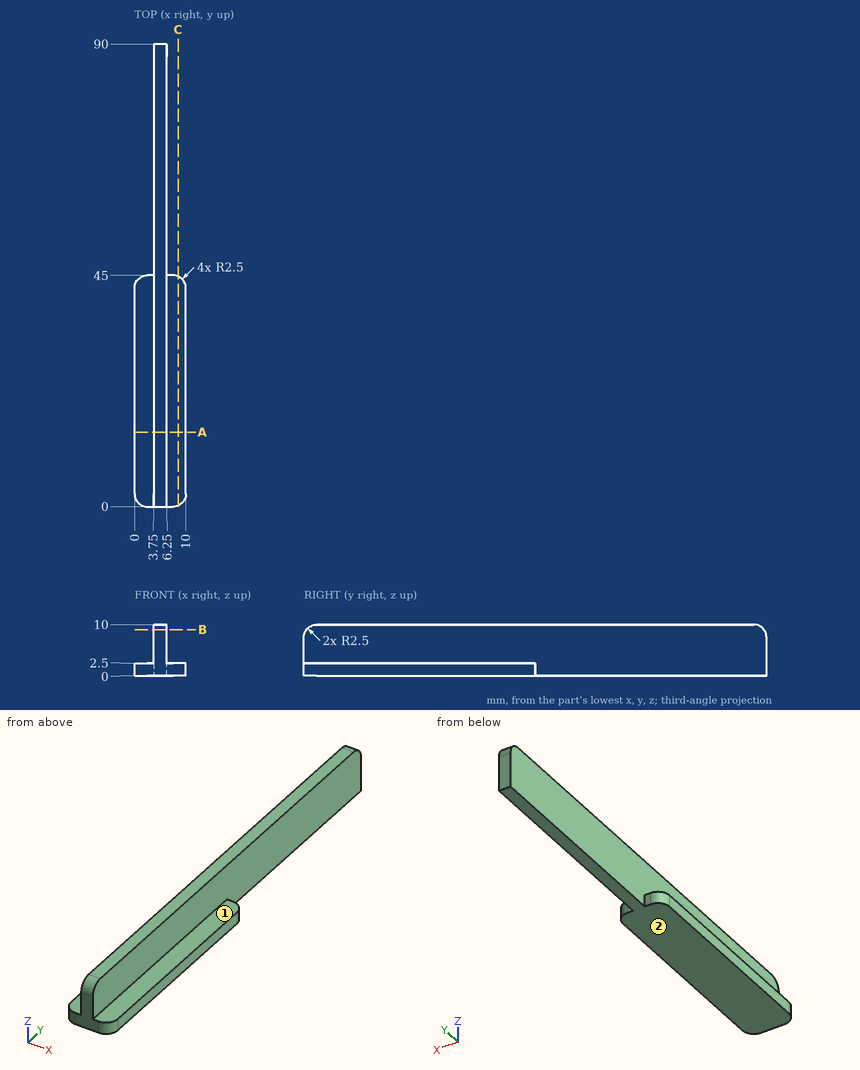
Geometry: see drawing. Coordinates: mm, zero at the bounding-box minimum. A direction names the side the tool comes from. Give positions to 0.01 mm unless a question says otherwise; leave off trailing zeros. Write each loop counter-clockwise with the first axis right and the second up, starting at its lowest first coordinate (ties: lowest second). Pieces come first, ordered by that corner, then holes. Notation, with made-up numbers: M -5.5,10 L 24.5,10 A26 cw 24.5,24 Z; hole C -8,55.25 d1. An arc over 180 degrees is marked long. Answer in a Markdown table with one row per item. Add a question column.
(1) Section B-B on z = 9. Return loops of the section in (x, y), and give its area (4 significant figures).
(2) Reachability of the marked faces 1 and 2 from +Z, -Z, +X, -X, +Y, -Y: full face, straight path, thin tool, end or side. Return the list, or none.
(3) Section C-C on x = 8.5. Return loops of the section in (y, z), and give its area (3 significant figures).
(4) First-contact query: pin 1 (1 mm diameter, centred on x = 3, z = 1, fed in from +Y); pin 2 (4 mm diameter, centred on x = 1.5, y = 12, fed in from +Z). Flat tips, straight axial feed; report the tip coordinate or a pass-through.
(5) Ray query, line 1 (X direction, y = 84, z = 2); line 2 (Y direction, x = 6, z = 8.5). Return the intervals inside material, ascending.
(6) Section A-A on y = 14.5. Return loops of the section in (x, z), and give its area (4 significant figures).
Result set:
| question | item | result |
|---|---|---|
| 1 | outline | M 3.75,0.5 L 6.25,0.5 L 6.25,89.5 L 3.75,89.5 Z |
| 1 | area | 222.5 mm^2 |
| 2 | face 1 | +Z, +X, +Y, -Y |
| 2 | face 2 | -Z, +X, -X, +Y, -Y |
| 3 | outline | M 0.21,0 L 44.79,0 L 44.79,2.5 L 0.21,2.5 Z |
| 3 | area | 111 mm^2 |
| 4 | pin 1 | stops at y = 45 |
| 4 | pin 2 | stops at z = 2.5 |
| 5 | line 1 | x = 3.75 to 6.25 |
| 5 | line 2 | y = 0.21 to 89.79 |
| 6 | outline | M 0,0 L 10,0 L 10,2.5 L 6.25,2.5 L 6.25,10 L 3.75,10 L 3.75,2.5 L 0,2.5 Z |
| 6 | area | 43.75 mm^2 |
